```python
from build123d import *

# Parameters (mm, degrees)
SKETCH1_W                = 381
SKETCH1_H                = 50.8
BOSS_EXTRUDE1_DEPTH      = 10
BOSS_EXTRUDE2_DEPTH      = 1.5875
BOSS_EXTRUDE2_DEPTH_BACK = 1.5875
SKETCH3_W                = 381
SKETCH3_H                = 50.8
CUT_EXTRUDE1_DEPTH       = 420.338538176


with BuildPart() as part:
    # Sketch1 → Boss-Extrude1 (new body)
    with BuildSketch(Plane(origin=(0, 0, 0), x_dir=(1, 0, 0), z_dir=(0, 1, 0))):
        with Locations((190.5, 25.4)):
            Rectangle(SKETCH1_W, SKETCH1_H)
    extrude(amount=BOSS_EXTRUDE1_DEPTH)

    # Sketch3 → Cut-Extrude1 (cut, through all)
    with BuildSketch(Plane(origin=(0, 10, 0), x_dir=(1, 0, 0), z_dir=(0, 1, 0))):
        with Locations((190.5, 25.4)):
            Rectangle(SKETCH3_W, SKETCH3_H)
    extrude(amount=-CUT_EXTRUDE1_DEPTH, mode=Mode.SUBTRACT)


with BuildPart() as body_2:
    # Sketch2 → Boss-Extrude2 (new, two sides: drawn at the far end of the back side and taken through both)
    with BuildSketch(Plane.XY.offset(-25.4).offset(-BOSS_EXTRUDE2_DEPTH_BACK)):
        Polygon((347.867965721, 10), (37.987965721, 10), (233.567965721, 177.64), (347.867965721, 177.64), align=None)
    extrude(amount=BOSS_EXTRUDE2_DEPTH + BOSS_EXTRUDE2_DEPTH_BACK)


solid = body_2.part
```
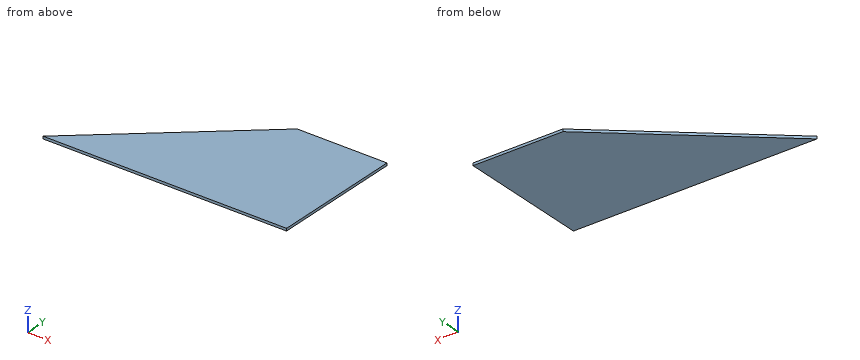
Build history of the part. All positions in model axes, mm. Give positions to 0.01 mm unless a question says otherwise; leave off trailing zeros. Loops run counter-clockwise (first coordinate to the right, second up) from the corner with the lowest first, then second, coordinate; pieces in that order, holes last. Notation, with made-up numbers: (25, 20.5) - (43, 20.5) arc R25 cw to (43, 55.5) - close; hole circle Ø4 at (4, 29). An arc over 180 degrees is marked (long way). Use a Markdown table: item, result.
(1) Band-saw the part on B-B (y = 58.5). Give the cut face in (x, z), and give its area (3 significant figures).
Taken from the geometry:
| item | result |
|---|---|
| outline | (94.57, -26.99) - (347.87, -26.99) - (347.87, -23.81) - (94.57, -23.81) - close |
| area | 804 mm2 |
(2) Band-saw the part on A-A (z = -25.25). Give the cut face in (x, y).
Taken from the geometry:
| item | result |
|---|---|
| outline | (37.99, 10) - (347.87, 10) - (347.87, 177.64) - (233.57, 177.64) - close |
(3) Wall check: line 1 along X through (y, z) = (170, -24.9); line 2 along X through (y, z) = (45, -26.4); line 3 along Y through (x, z) = (196, -26.75). Give the ranges that are in metal, low to high.
Taken from the geometry:
| item | result |
|---|---|
| line 1 | 224.65 to 347.87 |
| line 2 | 78.82 to 347.87 |
| line 3 | 10 to 145.44 |
